Autodesk Inventor part; units mm, degrees
ref_plane "YZ Plane" through (0, 0, 0) normal (1, 0, 0) x (0, 1, 0)
ref_plane "XZ Plane" through (0, 0, 0) normal (0, 1, 0) x (-1, 0, 0)
ref_plane "XY Plane" through (0, 0, 0) normal (0, 0, 1) x (1, 0, 0)
sketch "スケッチ1" plane through (0, 0, 0) normal (0, 0, 1) x (1, 0, 0)
  circle A0 centre (0, 5.8) radius 2.6
  circle A1 centre (0, 13.4) radius 2.6
  line L0 (-3.8, 0) -> (3.8, 0)
  line L1 (3.8, 0) -> (3.8, 17.6)
  line L2 (3.8, 17.6) -> (-3.8, 17.6)
  line L3 (-3.8, 17.6) -> (-3.8, 0)
  line L4 (-11.5586, 9.6) -> (11.5586, 9.6) construction
  point P0 (0, 0)
  point P1 (0, 0)
  point P2 (0, 9.6)
  dimension "LED_DIA" = 5.2
  dimension "d1" = 7.6
  dimension "LED_PITCH" = 7.6
  dimension "TOP_MARGIN" = 4.2
  dimension "BOTTOM_MARGIN" = 5.8
extrude "スペーサ" add sketch "スケッチ1" along normal blind 2
sketch "スケッチ2" plane through (0, 0, 0) normal (0, 0, -1) x (-1, 0, 0)
  line L0 (3.8, 17.6) -> (3.8, 0)
  line L1 (-3.8, 0) -> (-3.8, 17.6)
  line L2 (3.8, 0) -> (-3.8, 0)
  line L3 (-3.8, 0) -> (-3.8, 2)
  line L4 (-3.8, 2) -> (3.8, 2)
  line L5 (3.8, 2) -> (3.8, 0)
  line L6 (3.8, 10.2) -> (-3.8, 10.2)
  line L7 (-3.8, 10.2) -> (-3.8, 9)
  line L8 (-3.8, 9) -> (3.8, 9)
  line L9 (3.8, 9) -> (3.8, 10.2)
  circle A0 centre (0, 5.8) radius 2.9 construction
  circle A1 centre (0, 13.4) radius 2.9 construction
  circle A2 centre (0, 5.8) radius 2.6 construction
  circle A3 centre (0, 13.4) radius 2.6 construction
  line L10 (6.2058, 13.4) -> (-6.2058, 13.4) construction
  line L11 (-6.2058, 5.8) -> (6.2058, 5.8) construction
  line L12 (6.2058, 9.6) -> (-6.2058, 9.6) construction
  point P0 (0, 0)
  point P1 (3.8, 9.6)
  point P2 (-3.8, 9)
  point P3 (3.8, 9)
  point P4 (3.8, 10.2)
  point P5 (-3.8, 10.2)
  dimension "d8" = 5.8
  dimension "d9" = 2
  dimension "d10" = 1.2
extrude "押し出し2" add sketch "スケッチ2" along normal blind 2 contours L0 L8 L1 L6 | L0 L2 L1 L4
chamfer "面取り1" distance 0.6 angle 45 1 edges at (-2.6, 13.4, 2)
sketch "スケッチ3" plane through (-3.8, 0, 2) normal (0, -1, 0) x (1, 0, 0)
  line L0 (0, 0) -> (7.6, 0)
  line L1 (7.6, -4) -> (0, -4)
  line L2 (4.8, 0) -> (2.8, 0)
  line L3 (2.8, 0) -> (2.8, -4)
  line L4 (2.8, -4) -> (4.8, -4)
  line L5 (4.8, -4) -> (4.8, 0)
  point P0 (3.8, -2)
  point P1 (3.8, 0)
  dimension "d16" = 2
extrude "押し出し3" add sketch "スケッチ3" along normal blind 3
properties part number "LED-Spacer1"
Here's how the part is built. I have some questions about the finished solid (model axes, mm). A direction names the side the tool comes from. Coordinates: 2 decimals unless noted, no trailing zeros. Write each loop counter-clockwise with the first axis right and the second up, starting at its lowest first coordinate (ties: lowest second). Pieces come first, ordered by that corner, then holes. Notation, with made-up numbers: (-1, 22.5) - (32, 22.5) arc R34 cw to (32, 56.5) - close; hole circle Ø8 at (64.5, 36). An arc over 180 degrees is marked (long way). One line per item, written item: value.
1) On a 3-axis mill with a long thin cutter (end or side, diameter ignored), from which of +Z, -Z, +X, -X, +Y, -Y can I reach the whole of each face in a straight line? I mean faces 1 (the flat face through (-2, 0, 0)), 2 (the flat face through (-1, 3, 0)), 3 (the flat face through (-2, 16, 0)), 4 (the flat face through (2, 0, 0)). Say none if no direction works.
Model answer:
face 1: +Z, -Z, -X, -Y
face 2: -Z, +X, -X
face 3: -Z, +X, -X, +Y
face 4: +Z, -Z, +X, -Y
2) Suppose I cut it at A-A on y = 5.8. Write out the boundary of the cut face in (x, z), and give its area (3 significant figures).
Model answer:
outline: (-3.8, 0) - (-2.6, 0) - (-2.6, 2) - (-3.8, 2) - close; (2.6, 0) - (3.8, 0) - (3.8, 2) - (2.6, 2) - close
area: 4.80 mm²
3) Suppose I cut it at D-D on z = 0.8. Write out the boundary of the cut face in (x, y).
Model answer:
outline: (-3.8, 0) - (-1, 0) - (-1, -3) - (1, -3) - (1, 0) - (3.8, 0) - (3.8, 17.6) - (-3.8, 17.6) - close; hole circle Ø5.2 at (0, 5.8); hole circle Ø5.2 at (0, 13.4)
4) Suppose I cut it at C-C on z = -0.3. Write out the boundary of the cut face in (x, y), and give its area (3 significant figures).
Model answer:
outline: (-3.8, 0) - (-1, 0) - (-1, -3) - (1, -3) - (1, 0) - (3.8, 0) - (3.8, 2) - (-3.8, 2) - close; (-3.8, 9) - (3.8, 9) - (3.8, 10.2) - (-3.8, 10.2) - close
area: 30.3 mm²
5) Suppose I cut it at B-B on x = 0. Write out the boundary of the cut face in (y, z).
Model answer:
outline: (-3, -2) - (2, -2) - (2, 0) - (3.2, 0) - (3.2, 2) - (-3, 2) - close; (8.4, 0) - (9, 0) - (9, -2) - (10.2, -2) - (10.2, 0) - (10.8, 0) - (10.8, 1.4) - (10.2, 2) - (8.4, 2) - close; (16, 0) - (17.6, 0) - (17.6, 2) - (16.6, 2) - (16, 1.4) - close
6) I'm going to push flat-ended pins straight in: P1, Ø3, axis at x = -0.5, y = 6.5, coming from the +Z side; P2, Ø1.4, axis at x = -2.5, z = 0, coming from the -Y side; P3, Ø0.6, axis at x = 1, z = -1, coming from the +Y side. Where does each tip first touch, or does it pass through?
Model answer:
P1: passes through
P2: stops at y = 0
P3: stops at y = 10.2
7) We'd pull the mould along X, two halves only. Please class faces 5 (the flat face through (-1, -1, 0)), 6 (the cylindrical face through (-0.338, 3.222, 0.986)), 7 (the flat face through (0, 2, -1)): pulls with the +X half, pulls with the -X half, needs draft (parallel to the pull), parting line crosses it, or undercut.
Model answer:
face 5: pulls with the -X half
face 6: undercut
face 7: needs draft
8) I need wall thicknesses on line 1 along Y through (x, z) = (0, 0.9); line 2 along Y through (x, z) = (-0.25, -0.05); line 3 along Y through (x, z) = (-1.5, -0.75). Which ranges of each line are inside material? Lowest first, please.
Model answer:
line 1: y = -3 to 3.2, 8.4 to 10.8, 16 to 17.6
line 2: y = -3 to 2, 9 to 10.2
line 3: y = 0 to 2, 9 to 10.2
